Can you work these out from the model? Positions are in its coordinate system, mm. Round coordinates to 2 decimals unless told otherwise and drop trailing zeros. Return JSON: item names as keys, results as strings.
```python
from build123d import *

# Parameters (mm, degrees)
SKETCH_1_W                   = 12
SKETCH_1_H                   = 8
EXTRUDE_1_DEPTH              = 550
HOLE_WIZARD_M3_1_D           = 3.2
HOLE_WIZARD_M3_1_CBORE_D     = 6
HOLE_WIZARD_M3_1_CBORE_DEPTH = 3.4
PATTERN_LINEAR_1_COUNT       = 22
PATTERN_LINEAR_1_PITCH       = 25


with BuildPart() as part:
    # 草圖1 → 伸長1 (new body)
    with BuildSketch(Plane(origin=(0, 0, 0), x_dir=(0, 0, -1), z_dir=(1, 0, 0))):
        with Locations((0, 4)):
            Rectangle(SKETCH_1_W, SKETCH_1_H)
    extrude(amount=EXTRUDE_1_DEPTH)

    # M3 內六角圓柱頭螺釘的柱孔1 (through all)
    with Locations(Plane(origin=(10, 8, 0), x_dir=(0, 0, 1), z_dir=(0, 1, 0))):
        with Locations((0, 0)):
            hole_wizard_m3_1 = CounterBoreHole(HOLE_WIZARD_M3_1_D / 2, HOLE_WIZARD_M3_1_CBORE_D / 2, HOLE_WIZARD_M3_1_CBORE_DEPTH)

    # 直線複製排列1: M3 內六角圓柱頭螺釘的柱孔1 ×22
    with Locations(*[(i * PATTERN_LINEAR_1_PITCH, 0, 0) for i in range(1, PATTERN_LINEAR_1_COUNT)]):
        add(hole_wizard_m3_1, mode=Mode.SUBTRACT)


solid = part.part
```
Q1. If I drill on line 1 along Z through (x, y) = (410, 6.75); line 2 along Y through (x, z) = (35, -1.75); line 3 along Z through (x, y) = (210, 3.25), over which ranges is the centre line in solid material (lowest first)?
Results:
{"line 1": "z = -6 to -3, 3 to 6", "line 2": "y = 0 to 4.6", "line 3": "z = -6 to -1.6, 1.6 to 6"}
Q2. Suppose I cut it at A-A, the plane y = 6.75. State how many separate pieces and enclosed holes the cut face has, plus the area to 3 significant figures.
Results:
{"separate pieces": "1", "enclosed holes": "22", "area": "5,980 mm2"}
Q3. I'm going to push a flat-ended pin straight in: pin 1 Ø5 at (x, z) = (85, 0) entering from +Y. Where does the tip first touch, or does it pass through?
Results:
{"pin 1": "stops at y = 4.6"}
